```python
from build123d import *

# Parameters (mm, degrees)
BOSS_EXTRUDE1_DEPTH = 6.35
SKETCH2_R           = 1.95
SKETCH2_W           = 40.8
SKETCH2_H           = 20
CUT_EXTRUDE1_DEPTH  = 6.35


with BuildPart() as part:
    # Sketch1 → Boss-Extrude1 (new body)
    with BuildSketch(Plane.XY):
        Polygon((-30, -21.5), (-30, 21.5), (30, 21.5), (30, -21.5), (30, -27.85), (18, -27.85), (18, -21.5), (8, -21.5), (8, -27.85), (-8, -27.85), (-8, -21.5), (-18, -21.5), (-18, -27.85), (-30, -27.85), align=None)
    extrude(amount=BOSS_EXTRUDE1_DEPTH)

    # Sketch2 → Cut-Extrude1 (cut)
    with BuildSketch(Plane.XY.offset(6.35)):
        with Locations((-25.5, 16.3)):
            Circle(SKETCH2_R)
        with Locations((-25.5, 6.7)):
            Circle(SKETCH2_R)
        with Locations((25.5, 6.7)):
            Circle(SKETCH2_R)
        with Locations((25.5, 16.3)):
            Circle(SKETCH2_R)
        with Locations((0, 11.5)):
            Rectangle(SKETCH2_W, SKETCH2_H)
    extrude(amount=-CUT_EXTRUDE1_DEPTH, mode=Mode.SUBTRACT)


solid = part.part
```
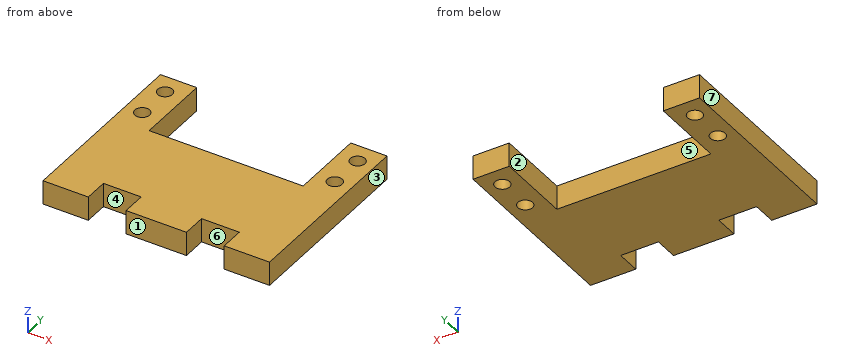
Check sheet for the modelled part. Datum: model origin and axes. Units: mm. Face numbers are marked on the shaded views. A direction names the side the tool comes from. Round coordinates to 2 decimals unless told otherwise and drop trailing zeros. Order: outer loops, then holes, each group sorted by start corner. A loop starts at its lowest first (then second) coordinate and runs counter-clockwise, first axis right, second up. Notation, with made-up numbers: (1.5, 75.25) - (7.5, 75.25) arc R22 ccw to (7.5, 91.25) - close; hole circle Ø8 at (76, 28). An arc over 180 degrees is marked (long way). Answer as CSV lines item,"result". Start each with the question number.
1) Section check D-D (z = 2). Record the cut outline in (x, y), then the cut area to 3 significant figures.
2) Section check B-B (x = -25.5). Record the cut outline in (y, z).
3) Tool access check on the marked faces 5, 6 and 7. Record the directions out of +Z, -Z, +X, -X, +Y, -Y that give a thin tool (end or side, any length) a straight path to the whole face; none if there is none.
4) Scan lines: probe 1 along Y at (x, z) = (25.5, 5); probe 2 along X at (y, z) = (-26, 1); probe 3 along X at (y, z) = (3.5, 1.5). Record each from-to range of solid material in increasing order.
5) Section check C-C (y = -24). Record the cut outline in (x, z).
6) Depth check by flat-ended pin: pin 1 (4 mm diameter, centred on x = -21.5, y = 7.5, fed in from -Z); pin 2 (3 mm diameter, centred on x = -25.5, y = 6.7, fed in from +Z); pin 3 (3 mm diameter, centred on x = -7, z = 2, fed in from +Y). Enter the tip coordinate at first touch or a pass-through.
7) Section check A-A (y = 10.5). Record the cut outline in (x, z), then the cut area to 3 significant figures.
8) Draft check along X on the marked faces 1, 2, 3 and 4. Enter one of: +X half, -X half, draft (parallel to the pull), parting line (faces both ways), or undercut.
Determined:
1,outline,"(-30, -27.85) - (-18, -27.85) - (-18, -21.5) - (-8, -21.5) - (-8, -27.85) - (8, -27.85) - (8, -21.5) - (18, -21.5) - (18, -27.85) - (30, -27.85) - (30, 21.5) - (20.4, 21.5) - (20.4, 1.5) - (-20.4, 1.5) - (-20.4, 21.5) - (-30, 21.5) - close; hole circle Ø3.9 at (-25.5, 6.7); hole circle Ø3.9 at (-25.5, 16.3); hole circle Ø3.9 at (25.5, 6.7); hole circle Ø3.9 at (25.5, 16.3)"
1,area,"1,970 mm^2"
2,outline,"(-27.85, 0) - (4.75, 0) - (4.75, 6.35) - (-27.85, 6.35) - close; (8.65, 0) - (14.35, 0) - (14.35, 6.35) - (8.65, 6.35) - close; (18.25, 0) - (21.5, 0) - (21.5, 6.35) - (18.25, 6.35) - close"
3,face 5,"+Z, -Z, +Y"
3,face 6,"+Z, -Z, -Y"
3,face 7,"+Z, -Z, -X, +Y, -Y"
4,probe 1,"-27.85 to 4.75, 8.65 to 14.35, 18.25 to 21.5"
4,probe 2,"-30 to -18, -8 to 8, 18 to 30"
4,probe 3,"-30 to -20.4, 20.4 to 30"
5,outline,"(-30, 0) - (-18, 0) - (-18, 6.35) - (-30, 6.35) - close; (-8, 0) - (8, 0) - (8, 6.35) - (-8, 6.35) - close; (18, 0) - (30, 0) - (30, 6.35) - (18, 6.35) - close"
6,pin 1,"z = 0"
6,pin 2,"through"
6,pin 3,"y = 1.5"
7,outline,"(-30, 0) - (-20.4, 0) - (-20.4, 6.35) - (-30, 6.35) - close; (20.4, 0) - (30, 0) - (30, 6.35) - (20.4, 6.35) - close"
7,area,"122 mm^2"
8,face 1,"draft"
8,face 2,"undercut"
8,face 3,"+X half"
8,face 4,"undercut"
